```python
from build123d import *

# Parameters (mm, degrees)
EXTRUDE_5_DEPTH      = 30
EXTRUDE_5_DEPTH_BACK = 30
F_1_FR_R             = 5
EXTRUDE_6_DEPTH      = 20
EXTRUDE_6_DEPTH_BACK = 20


with BuildPart() as part:
    # Эскиз1_fr → Бобышка-Вытянуть5 (new, two sides: drawn at the far end of the back side and taken through both)
    with BuildSketch(Plane.XY.offset(-EXTRUDE_5_DEPTH_BACK)):
        with BuildLine():
            Line((-5.557606452, -13.932444528), (-5.557606452, -62.642280008))
            Line((-5.557606452, -62.642280008), (5.557606452, -62.642280008))
            Line((5.557606452, -62.642280008), (5.557606452, -13.932444528))
            ThreePointArc((5.557606452, -13.932444528), (0, 15), (-5.557606452, -13.932444528))
        make_face()
        Circle(F_1_FR_R, mode=Mode.SUBTRACT)
    extrude(amount=EXTRUDE_5_DEPTH + EXTRUDE_5_DEPTH_BACK)


with BuildPart() as body_2:
    # Эскиз3 → Бобышка-Вытянуть6 (new, two sides: drawn at the far end of the back side and taken through both)
    with BuildSketch(Plane(origin=(0, 0, 0), x_dir=(0, 0, -1), z_dir=(1, 0, 0)).offset(-EXTRUDE_6_DEPTH_BACK)):
        Polygon((-58.394498043, -50.25314581), (-85.938130262, -50.25314581), (-85.938130262, 27.580465306), (-80.938130262, 27.580465306), (-80.938130262, -45.25314581), (-63.394498043, -45.25314581), (-63.394498043, 27.580465306), (-58.394498043, 27.580465306), align=None)
    extrude(amount=EXTRUDE_6_DEPTH + EXTRUDE_6_DEPTH_BACK)


with BuildPart() as body_2_1:
    # Move Body 1: moved
    add(body_2.part.moved(Location((0, 0, -70))))


with BuildPart() as part_1:
    add(part.part)

    # Combine 1: union body 2
    add(body_2_1.part)


solid = part_1.part
```
Here's how the part is built. I have some questions about the finished solid (model axes, mm). A direction names the side the tool comes from. Coordinates: 2 decimals unless noted, no trailing zeros. Loops run counter-clockwise (first coordinate to the right, second up) from the corner with the lowest first, then second, coordinate; pieces in that order, holes last. Notation, with made-up numbers: (68.5, -37) - (117.5, -37) arc R19 ccw to (117.5, -14) - close; hole circle Ø2 at (44, 10). An arc over 180 degrees is marked (long way). Answer as CSV lines item,"result".
Q1. If we section it at A-A, the plane x = 0: Write out the boundary of the cut face in (y, z), and give its area (3 significant figures).
Response:
outline,"(-62.64, -30) - (-5, -30) - (-5, -11.61) - (5, -11.61) - (5, -30) - (15, -30) - (15, -11.61) - (27.58, -11.61) - (27.58, -6.61) - (15, -6.61) - (15, 10.94) - (27.58, 10.94) - (27.58, 15.94) - (15, 15.94) - (15, 30) - (5, 30) - (5, 15.94) - (-5, 15.94) - (-5, 30) - (-62.64, 30) - close; hole (-5, -6.61) - (5, -6.61) - (5, 10.94) - (-5, 10.94) - close"
area,"4,280 mm2"
Q2. If we section it at D-D, the plane y = -34.5: Write out the boundary of the cut face in (x, z), and give its area (3 significant figures).
Response:
outline,"(-20, -11.61) - (-5.56, -11.61) - (-5.56, -30) - (5.56, -30) - (5.56, -11.61) - (20, -11.61) - (20, -6.61) - (5.56, -6.61) - (5.56, 10.94) - (20, 10.94) - (20, 15.94) - (5.56, 15.94) - (5.56, 30) - (-5.56, 30) - (-5.56, 15.94) - (-20, 15.94) - (-20, 10.94) - (-5.56, 10.94) - (-5.56, -6.61) - (-20, -6.61) - close"
area,"956 mm2"
Q3. For pin 1 (3 mm diameter, centred on x = 0.5, y = -2.5, fed in from -Z); pin 2 (16 mm diameter, centred on x = 16, z = -3.5, fed in from -Y); pin 3 (9 mm diameter, centred on y = -25, z = 2.5, fed in from +X), each with a flat end and sliding along its axis, tell me the tip position at first contact or that it passes through.
Response:
pin 1,"z = -11.61"
pin 2,"y = -50.25"
pin 3,"x = 5.56"
Q4. For faces 5 (the face through (0.58, 14.99, -20.93)), 6 (the face through (-13, -45.253, 2)), 7 (the face through (13, -50.253, 2)), 8 (the face through (-9, -16, 10.938)), which set-ups out of +Z, -Z, +X, -X, +Y, -Y let a thin tool reach every point of the face, with its end or its side?
Response:
face 5,"-Z"
face 6,"-X"
face 7,"+Z, -Z, +X, -Y"
face 8,"none"
Q5. We'd pull the mould along Z, two halves only. Please class faces 1 (the face through (-5.558, -43, -14)), 2 (the face through (5.558, -30, 2)), 3 (the face through (-9, -21, 15.938)), 4 (the face through (0, -15, -30)): pulls with the +Z half, pulls with the -Z half, needs draft (parallel to the pull), parting line crosses it, or undercut.
Response:
face 1,"needs draft"
face 2,"undercut"
face 3,"pulls with the +Z half"
face 4,"pulls with the -Z half"
Q6. If we section it at C-C, the plane z = 6.5: Write out the boundary of the cut face in (x, y), and give its area (3 significant figures).
Response:
outline,"(-20, -50.25) - (-5.56, -50.25) - (-5.56, -62.64) - (5.56, -62.64) - (5.56, -50.25) - (20, -50.25) - (20, -45.25) - (5.56, -45.25) - (5.56, -13.93) arc R15 ccw (long way) to (-5.56, -13.93) - (-5.56, -45.25) - (-20, -45.25) - close; hole circle Ø10 at (0, 0)"
area,"1,310 mm2"
Q7. If I drill on L1, parallel to Y at x = 0, z = 26.5; L2, parallel to X at y = 0, z = 24.75; L3, parallel to Z at x = 18.5, y = 2.5, over which ranges is the centre line in solid material (lowest first)? Write a range as [from, to].
Response:
L1,"[-62.64, -5], [5, 15]"
L2,"[-15, -5], [5, 15]"
L3,"[-11.61, -6.61], [10.94, 15.94]"
